Part model, mm, in its own coordinate system. Face numbers are marked on the shaded views. A direction names the side the tool comes from. Round coordinates to 2 decimals unless told otherwise and drop trailing zeros. Write each loop counter-clockwise with the first axis right and the second up, starting at its lowest first coordinate (ties: lowest second). Pieces come first, ordered by that corner, then holes. Notation, with made-up numbers: (-36, 84) -> (-15, 84) arc R27 ccw to (-15, 121) -> close; hole circle Ø4 at (-13, 15.25). An arc over 180 degrees is marked (long way). Use CSV: the item, a comma, the result in double quotes. Start each with the question number.
(1) Probe line 1 (Y direction, x = 6, z = 20); line 2 (X direction, y = 0.25, z = 14); line 3 (Z direction, x = -7.5, y = 1.75). List the from-to ranges inside material, lowest first. Write a range as [from, to].
(2) Saw through at A-A (z = 19.75). Give the cut face in (x, y), plus the area to 3 significant figures.
(3) Saw through at C-C (y = -6). Give the cut face in (x, z), plus the area to 3 significant figures.
(4) Drop flat-ended pins along their axis: pin 1 (2 mm diameter, centred on x = -1.5, y = 1, fed in from +Z); pin 2 (4.5 mm diameter, centred on x = -6, y = -6, fed in from +Z); pin 3 (0.8 mm diameter, centred on x = -6, y = 6, fed in from +Z). Give the stop position or say it passes through.
(5) Saw through at B-B (x = 0.75). Give the cut face in (y, z), plus the area to 4 significant figures.
(6) Two-plate mould, pull along X, no slides. Class the marked faces 1, 2, 3 and 4: released by +X, released by -X, zero draft, split by the parting line, or undercut.
(7) Saw through at D-D (z = 6.75). Give the cut face in (x, y), plus the area to 3 significant figures.
(8) Which spindle directions (+Z, -Z, +X, -X, +Y, -Y) get a long thin tool onto all of the face, cutting with end or side? Do the marked faces 5 and 6. Say none if no direction does.
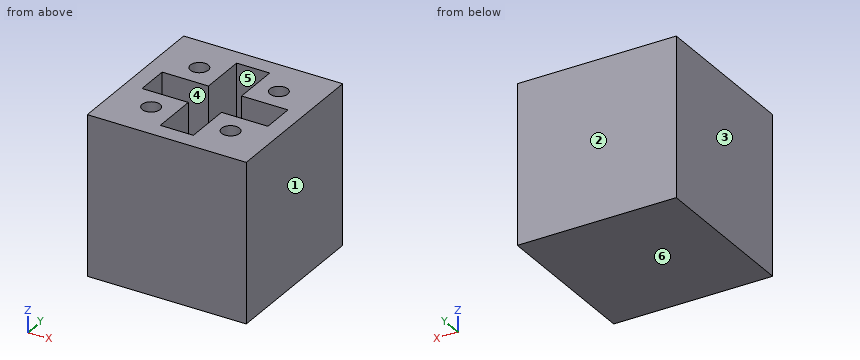
```python
from build123d import *

# Parameters (mm, degrees)
F0_W     = 24
F0_H     = 24
F0_W_2   = 7
F0_H_2   = 7
F0_R     = 1.35
F1_DEPTH = 24
F2_T     = -2.5
F3_DEPTH = 24
F4_DEPTH = 13


with BuildPart() as f1:
    # F0 (on Top) → F1 (new body)
    with BuildSketch(Plane.XY):
        Rectangle(F0_W, F0_H)
        with Locations((-6, -6)):
            Rectangle(F0_W_2, F0_H_2, mode=Mode.SUBTRACT)
        with Locations((6, -6)):
            Rectangle(F0_W_2, F0_H_2, mode=Mode.SUBTRACT)
        with Locations((-6, 6)):
            Rectangle(F0_W_2, F0_H_2, mode=Mode.SUBTRACT)
        with Locations((6, 6)):
            Rectangle(F0_W_2, F0_H_2, mode=Mode.SUBTRACT)
        with Locations((-6, 6)):
            Rectangle(F0_W_2, F0_H_2)
        with Locations((-6, 6)):
            Circle(F0_R, mode=Mode.SUBTRACT)
        with Locations((-6, 6)):
            Circle(F0_R)
        with Locations((6, 6)):
            Rectangle(F0_W_2, F0_H_2)
        with Locations((6, 6)):
            Circle(F0_R, mode=Mode.SUBTRACT)
        with Locations((6, 6)):
            Circle(F0_R)
        with Locations((6, -6)):
            Rectangle(F0_W_2, F0_H_2)
        with Locations((6, -6)):
            Circle(F0_R, mode=Mode.SUBTRACT)
        with Locations((6, -6)):
            Circle(F0_R)
        with Locations((-6, -6)):
            Rectangle(F0_W_2, F0_H_2)
        with Locations((-6, -6)):
            Circle(F0_R, mode=Mode.SUBTRACT)
        with Locations((-6, -6)):
            Circle(F0_R)
    extrude(amount=F1_DEPTH)

    # F2
    f2_openings = [f1.faces().sort_by_distance(p)[0] for p in [
        (0, 0, 24),
    ]]
    offset(amount=F2_T, openings=f2_openings)

    # F0 (on Top) → F3 (join)
    with BuildSketch(Plane.XY):
        with Locations((-6, 6)):
            Rectangle(F0_W_2, F0_H_2)
        with Locations((-6, 6)):
            Circle(F0_R, mode=Mode.SUBTRACT)
        with Locations((-6, -6)):
            Rectangle(F0_W_2, F0_H_2)
        with Locations((-6, -6)):
            Circle(F0_R, mode=Mode.SUBTRACT)
        with Locations((6, -6)):
            Rectangle(F0_W_2, F0_H_2)
        with Locations((6, -6)):
            Circle(F0_R, mode=Mode.SUBTRACT)
        with Locations((6, 6)):
            Rectangle(F0_W_2, F0_H_2)
        with Locations((6, 6)):
            Circle(F0_R, mode=Mode.SUBTRACT)
    extrude(amount=F3_DEPTH)

    # F0 (on Top) → F4 (join)
    with BuildSketch(Plane.XY):
        with Locations((-6, 6)):
            Circle(F0_R)
        with Locations((-6, -6)):
            Circle(F0_R)
        with Locations((6, -6)):
            Circle(F0_R)
        with Locations((6, 6)):
            Circle(F0_R)
    extrude(amount=F4_DEPTH)


solid = f1.part
```
Answers:
1,line 1,"y = [-12, -7.35], [-4.65, -2.5], [2.5, 4.65], [7.35, 12]"
1,line 2,"x = [-12, -9.5], [9.5, 12]"
1,line 3,"z = [0, 2.5]"
2,outline,"(-12, -12) -> (12, -12) -> (12, 12) -> (-12, 12) -> close; hole (-9.5, -2.5) -> (-2.5, -2.5) -> (-2.5, -9.5) -> (2.5, -9.5) -> (2.5, -2.5) -> (9.5, -2.5) -> (9.5, 2.5) -> (2.5, 2.5) -> (2.5, 9.5) -> (-2.5, 9.5) -> (-2.5, 2.5) -> (-9.5, 2.5) -> close; hole circle Ø2.7 at (-6, -6); hole circle Ø2.7 at (-6, 6); hole circle Ø2.7 at (6, -6); hole circle Ø2.7 at (6, 6)"
2,area,"388 mm²"
3,outline,"(-12, 0) -> (12, 0) -> (12, 24) -> (7.35, 24) -> (7.35, 13) -> (4.65, 13) -> (4.65, 24) -> (2.5, 24) -> (2.5, 2.5) -> (-2.5, 2.5) -> (-2.5, 24) -> (-4.65, 24) -> (-4.65, 13) -> (-7.35, 13) -> (-7.35, 24) -> (-12, 24) -> close"
3,area,"409 mm²"
4,pin 1,"stops at z = 2.5"
4,pin 2,"stops at z = 24"
4,pin 3,"stops at z = 13"
5,outline,"(-12, 0) -> (12, 0) -> (12, 24) -> (9.5, 24) -> (9.5, 2.5) -> (-9.5, 2.5) -> (-9.5, 24) -> (-12, 24) -> close"
5,area,"167.5 mm²"
6,face 1,"released by +X"
6,face 2,"zero draft"
6,face 3,"released by -X"
6,face 4,"undercut"
7,outline,"(-12, -12) -> (12, -12) -> (12, 12) -> (-12, 12) -> close; hole (-9.5, -2.5) -> (-2.5, -2.5) -> (-2.5, -9.5) -> (2.5, -9.5) -> (2.5, -2.5) -> (9.5, -2.5) -> (9.5, 2.5) -> (2.5, 2.5) -> (2.5, 9.5) -> (-2.5, 9.5) -> (-2.5, 2.5) -> (-9.5, 2.5) -> close"
7,area,"411 mm²"
8,face 5,"+Z"
8,face 6,"-Z, +X, -X, +Y, -Y"
